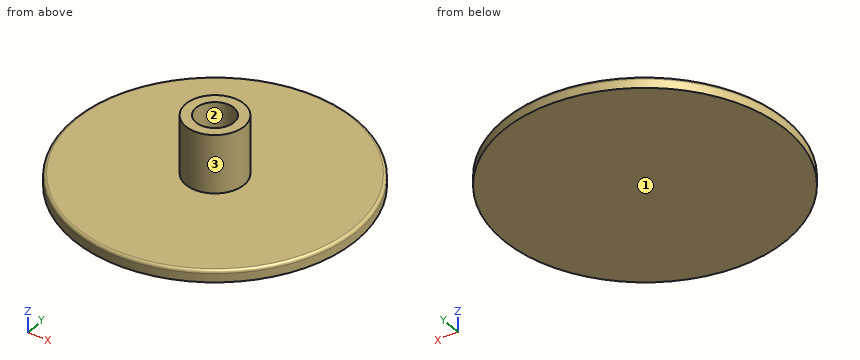
```python
from build123d import *

# Parameters (mm, degrees)
SKETCH_R     = 12.15
PAD_DEPTH    = 1
FILLET_R     = 0.25
SKETCH001_R  = 2.5
PAD001_DEPTH = 5
SKETCH002_R  = 1.625
POCKET_DEPTH = 5


with BuildPart() as part:
    # Sketch → Pad (new body)
    with BuildSketch(Plane.XY):
        Circle(SKETCH_R)
    extrude(amount=PAD_DEPTH)

    # Fillet
    fillet_edges = [part.edges().sort_by_distance(p)[0] for p in [
        (-12.15, 0, 1),
    ]]
    fillet(fillet_edges, radius=FILLET_R)

    # Sketch001 (on Face4 of Fillet) → Pad001 (join)
    with BuildSketch(Plane.XY.offset(1)):
        Circle(SKETCH001_R)
    extrude(amount=PAD001_DEPTH)

    # Sketch002 (on Face6 of Pad001) → Pocket (cut)
    with BuildSketch(Plane.XY.offset(6)):
        Circle(SKETCH002_R)
    extrude(amount=-POCKET_DEPTH, mode=Mode.SUBTRACT)


solid = part.part
```
CAD build for the part. Positions are in the model's coordinates, mm. Face numbers are marked on the shaded views. Round coordinates to 2 decimals unless told otherwise and drop trailing zeros. Loops run counter-clockwise (first coordinate to the right, second up) from the corner with the lowest first, then second, coordinate; pieces in that order, holes last. Notation, with made-up numbers: M -31.5,-13.5 L 16.5,-13.5 A19 ccw 16.5,0.5 Z; hole C 79.25,-14 d10. An arc over 180 degrees is marked long. Use a Markdown table: item, result. Add a question column.
(1) Drill centre lines: line 1 (Y direction, x = 0, z = 4.45) (3 decimals); line 2 (Z direction, x = -11, y = -2.5); line 3 (X direction, y = -1.75, z = 0.4). Where is each one in solid material? Low to high.
(2) Cut at C-C (z = 5). Give the cut face in (x, y) (3 decimals), and give its area (3 significant figures).
(3) Pull direction X, two halves, no side cores. Call the marked faces 1, 2 and 3: +X half, -X half, draft (parallel to the pull), parting line (faces both ways), or undercut.
(4) Flat gauge pins, fed straight in: pin 1 (3 mm diameter, centred on x = 0, y = 0, fed in from +Z); pin 2 (1 mm diameter, centred on y = 8, z = 1, fed in from -X). Where does each tip first touch, or does it go through?
(5) Cut at A-A (x = 0). Give the cut face in (y, z) (3 decimals).
Geometry says:
| question | item | result |
|---|---|---|
| 1 | line 1 | y = -2.5 to -1.625, 1.625 to 2.5 |
| 1 | line 2 | z = 0 to 1 |
| 1 | line 3 | x = -12.02 to 12.02 |
| 2 | outline | C 0,0 d5; hole C 0,0 d3.25 |
| 2 | area | 11.3 mm² |
| 3 | face 1 | draft |
| 3 | face 2 | undercut |
| 3 | face 3 | parting line |
| 4 | pin 1 | stops at z = 1 |
| 4 | pin 2 | stops at x = -9.52 |
| 5 | outline | M -12.15,0 L 12.15,0 L 12.15,0.75 A0.25 ccw 11.9,1 L 2.5,1 L 2.5,6 L 1.625,6 L 1.625,1 L -1.625,1 L -1.625,6 L -2.5,6 L -2.5,1 L -11.9,1 A0.25 ccw -12.15,0.75 Z |
